```python
from build123d import *

# Parameters (mm, degrees)
SKETCH1_R           = 1.5
SKETCH1_R_2         = 2
SKETCH1_R_3         = 2.5
SKETCH1_R_4         = 3.96875
BOSS_EXTRUDE1_DEPTH = 3.175
CUT_EXTRUDE1_START  = -3.175
SKETCH2_R           = 3.96875
SKETCH2_R_2         = 1.5
SKETCH2_R_3         = 2
SKETCH2_R_4         = 2.5
CUT_EXTRUDE1_DEPTH  = 3.175


with BuildPart() as part:
    # Sketch1 → Boss-Extrude1 (new body)
    with BuildSketch(Plane(origin=(0, 0, 0), x_dir=(1, 0, 0), z_dir=(0, 1, 0))):
        Polygon((240.38814, 0), (225.38814, 25.980762114), (45, 25.980762114), (135.19407, 182.201473895), (120.19407, 208.182236008), (90.19407, 208.182236008), (0, 51.961524227), (-90.19407, 208.182236008), (-120.19407, 208.182236008), (-135.19407, 182.201473895), (-45, 25.980762114), (-225.38814, 25.980762114), (-240.38814, 0), (-225.38814, -25.980762114), (-45, -25.980762114), (-135.19407, -182.201473895), (-120.19407, -208.182236008), (-90.19407, -208.182236008), (0, -51.961524227), (90.19407, -208.182236008), (120.19407, -208.182236008), (135.19407, -182.201473895), (45, -25.980762114), (225.38814, -25.980762114), align=None)
        with Locations(Location((208.18221, 0, 0), (0, 0, 270))):
            Circle(SKETCH1_R, mode=Mode.SUBTRACT)
        with Locations(Location((104.091105, -180.291082476, 0), (0, 0, 270))):
            Circle(SKETCH1_R, mode=Mode.SUBTRACT)
        with Locations(Location((-104.091105, -180.291082476, 0), (0, 0, 270))):
            Circle(SKETCH1_R, mode=Mode.SUBTRACT)
        with Locations(Location((-208.18221, 0, 0), (0, 0, 270))):
            Circle(SKETCH1_R, mode=Mode.SUBTRACT)
        with Locations(Location((-104.091105, 180.291082476, 0), (0, 0, 270))):
            Circle(SKETCH1_R, mode=Mode.SUBTRACT)
        with Locations(Location((104.091105, 180.291082476, 0), (0, 0, 270))):
            Circle(SKETCH1_R, mode=Mode.SUBTRACT)
        with Locations(Location((16.497783942, 9.525, 0), (0, 0, 270))):
            Circle(SKETCH1_R_2, mode=Mode.SUBTRACT)
        with Locations(Location((0, -19.05, 0), (0, 0, 270))):
            Circle(SKETCH1_R_2, mode=Mode.SUBTRACT)
        with Locations(Location((-16.497783942, 9.525, 0), (0, 0, 270))):
            Circle(SKETCH1_R_2, mode=Mode.SUBTRACT)
        with Locations(Location((32.066865, 55.541439419, 0), (0, 0, 270))):
            Circle(SKETCH1_R_3, mode=Mode.SUBTRACT)
        with Locations(Location((64.13373, 0, 0), (0, 0, 270))):
            Circle(SKETCH1_R_3, mode=Mode.SUBTRACT)
        with Locations(Location((32.066865, -55.541439419, 0), (0, 0, 270))):
            Circle(SKETCH1_R_3, mode=Mode.SUBTRACT)
        with Locations(Location((-32.066865, -55.541439419, 0), (0, 0, 270))):
            Circle(SKETCH1_R_3, mode=Mode.SUBTRACT)
        with Locations(Location((-64.13373, 0, 0), (0, 0, 270))):
            Circle(SKETCH1_R_3, mode=Mode.SUBTRACT)
        with Locations(Location((-32.066865, 55.541439419, 0), (0, 0, 270))):
            Circle(SKETCH1_R_3, mode=Mode.SUBTRACT)
        with Locations(Location((0, 0, 0), (0, 0, 270))):
            Circle(SKETCH1_R_4, mode=Mode.SUBTRACT)
    extrude(amount=BOSS_EXTRUDE1_DEPTH)

    # Sketch2 → Cut-Extrude1 (cut)
    # profile 1 of 3: a face of its own
    with BuildSketch(Plane(origin=(0, 3.175, 0), x_dir=(1, 0, 0), z_dir=(0, 1, 0)).offset(CUT_EXTRUDE1_START)):
        with BuildLine():
            ThreePointArc((228.675327889, -132.025762114), (-228.675327889, -132.025762114), (0, 264.051524227))
            Line((0, 264.051524227), (0, 51.961524227))
            Line((0, 51.961524227), (-90.19407, 208.182236008))
            Line((-90.19407, 208.182236008), (-120.19407, 208.182236008))
            Line((-120.19407, 208.182236008), (-135.19407, 182.201473895))
            Line((-135.19407, 182.201473895), (-45, 25.980762114))
            Line((-45, 25.980762114), (-225.38814, 25.980762114))
            Line((-225.38814, 25.980762114), (-240.38814, 0))
            Line((-240.38814, 0), (-225.38814, -25.980762114))
            Line((-225.38814, -25.980762114), (-45, -25.980762114))
            Line((-45, -25.980762114), (-135.19407, -182.201473895))
            Line((-135.19407, -182.201473895), (-120.19407, -208.182236008))
            Line((-120.19407, -208.182236008), (-90.19407, -208.182236008))
            Line((-90.19407, -208.182236008), (0, -51.961524227))
            Line((0, -51.961524227), (90.19407, -208.182236008))
            Line((90.19407, -208.182236008), (120.19407, -208.182236008))
            Line((120.19407, -208.182236008), (135.19407, -182.201473895))
            Line((135.19407, -182.201473895), (45, -25.980762114))
            Line((45, -25.980762114), (228.675327889, -132.025762114))
        make_face()
    # profile 2 of 3: a face of its own
    with BuildSketch(Plane(origin=(0, 3.175, 0), x_dir=(1, 0, 0), z_dir=(0, 1, 0)).offset(CUT_EXTRUDE1_START)):
        Circle(SKETCH2_R)
    # profile 3 of 3: a face of its own
    with BuildSketch(Plane(origin=(0, 3.175, 0), x_dir=(1, 0, 0), z_dir=(0, 1, 0)).offset(CUT_EXTRUDE1_START)):
        Polygon((0, 0), (45, -25.980762114), (135.19407, -182.201473895), (120.19407, -208.182236008), (90.19407, -208.182236008), (0, -51.961524227), (-90.19407, -208.182236008), (-120.19407, -208.182236008), (-135.19407, -182.201473895), (-45, -25.980762114), (-225.38814, -25.980762114), (-240.38814, 0), (-225.38814, 25.980762114), (-45, 25.980762114), (-135.19407, 182.201473895), (-120.19407, 208.182236008), (-90.19407, 208.182236008), (0, 51.961524227), align=None)
        with Locations((104.091105, -180.291082476)):
            Circle(SKETCH2_R_2, mode=Mode.SUBTRACT)
        with Locations((-208.18221, 0)):
            Circle(SKETCH2_R_2, mode=Mode.SUBTRACT)
        with Locations((-104.091105, 180.291082476)):
            Circle(SKETCH2_R_2, mode=Mode.SUBTRACT)
        with Locations((-16.497783942, 9.525)):
            Circle(SKETCH2_R_3, mode=Mode.SUBTRACT)
        with Locations((0, -19.05)):
            Circle(SKETCH2_R_3, mode=Mode.SUBTRACT)
        with Locations((-32.066865, 55.541439419)):
            Circle(SKETCH2_R_4, mode=Mode.SUBTRACT)
        with Locations((-64.13373, 0)):
            Circle(SKETCH2_R_4, mode=Mode.SUBTRACT)
        with Locations((-32.066865, -55.541439419)):
            Circle(SKETCH2_R_4, mode=Mode.SUBTRACT)
        with Locations((-104.091105, -180.291082476)):
            Circle(SKETCH2_R_2, mode=Mode.SUBTRACT)
        with Locations((32.066865, -55.541439419)):
            Circle(SKETCH2_R_4, mode=Mode.SUBTRACT)
    extrude(amount=CUT_EXTRUDE1_DEPTH, mode=Mode.SUBTRACT)


solid = part.part
```
Geometry check sheet. Reference: the model listing, model coordinates, mm. A direction names the side the tool comes from. Give positions to 0.01 mm unless a question says otherwise; leave off trailing zeros. Order: outer loops, then holes, each group sorted by start corner. A loop starts at its lowest first (then second) coordinate and runs counter-clockwise, first axis right, second up. Notation, with made-up numbers: (30.5, -0.5) - (63.5, -0.5) arc R17 cw to (63.5, 22.5) - close; hole circle Ø1 at (47, 52.25). An arc over 180 degrees is marked (long way). Write item = value, one per line. Start each with the question number.
1) Section check C-C (z = 7.5). Enter the section's corners in (x, y) (3 decimals).
2) Access from +Z, -Z, +X, -X, +Y, -Y to the whole of each face (thin tool, end or side, straight path). Record for faces 1 (the flat face through (23.9, 1.6, 13.8)), 2 (the flat face through (89.466, 1.565, -102.998)).
3) Section check B-B (x = 196). Enter the section's corners in (y, z) (3 decimals), then the cut area to 3 significant figures.
4) Gauge pin test, flat end, axial feed: pin 1 Ø3 at (x, z) = (16.5, -9.52) entering from -Y. Record the tip position at first contact, or that the pin passes through.
5) Scan lines: L1, parallel to X at y = 1, z = 0; L2, parallel to Z at x = 103, y = 2.5; L3, parallel to Z at x = 173.5, y = 0.2. Record each from-to range of solid material in increasing order.
6) Section check A-A (y = 0.8). Enter the section's corners in (x, z) (1 decimal), then the cut area to 3 significant figures.
Geometry check:
q1.outline = (12.99, 0) - (236.058, 0) - (236.058, 3.175) - (12.99, 3.175) - close
q2.face_1 = +Z, -X, +Y, -Y
q2.face_2 = +X, +Y, -Y
q3.outline = (0, -25.981) - (3.175, -25.981) - (3.175, 25.981) - (0, 25.981) - close
q3.area = 165 mm2
q4.pin_1 = through
q5.L1 = 3.97 to 61.63, 66.63 to 206.68, 209.68 to 240.39
q5.L2 = -208.18 to -181.32, -179.26 to -126.44, -25.98 to 25.98
q5.L3 = -25.98 to 25.98
q6.outline = (0, -52) - (90.2, -208.2) - (120.2, -208.2) - (135.2, -182.2) - (45, -26) - (225.4, -26) - (240.4, 0) - (225.4, 26) - (45, 26) - (3.4, 2) arc R4 cw to (0, -4) - close; hole circle Ø4 at (16.5, -9.5); hole circle Ø5 at (32.1, -55.5); hole circle Ø5 at (64.1, 0); hole circle Ø3 at (104.1, -180.3); hole circle Ø3 at (208.2, 0)
q6.area = 21,800 mm2
